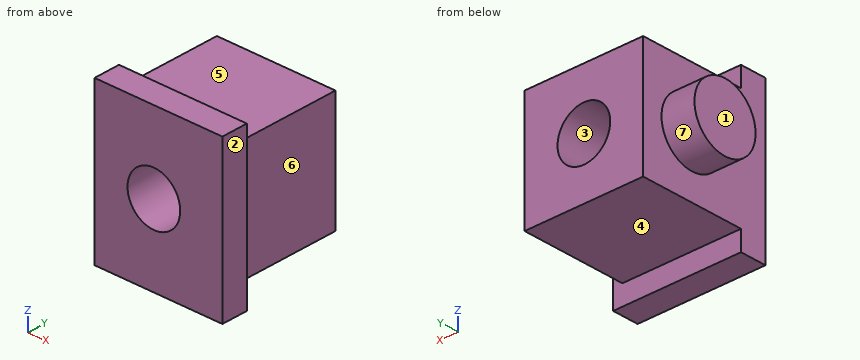
Autodesk Inventor part; units mm, degrees
ref_plane "YZ Plane" through (0, 0, 0) normal (1, 0, 0) x (0, 1, 0)
ref_plane "XZ Plane" through (0, 0, 0) normal (0, 1, 0) x (-1, 0, 0)
ref_plane "XY Plane" through (0, 0, 0) normal (0, 0, 1) x (1, 0, 0)
sketch "Sketch1" plane through (0, 0, 0) normal (0, 1, 0) x (-1, 0, 0)
  line L0 (0, 0) -> (30.1625, 0)
  line L1 (30.1625, 0) -> (30.1625, -31.75)
  line L2 (30.1625, -31.75) -> (0, -31.75)
  line L3 (0, -31.75) -> (0, 0)
  dimension "d0" = 31.75
  dimension "d1" = 30.1625
extrude "Extrusion1" add sketch "Sketch1" along normal blind 31.75
sketch "Sketch2" plane through (-30.1625, 0, 0) normal (0, 0, 1) x (1, 0, 0)
  line L0 (0, 0) -> (0, 31.75)
  line L1 (30.1625, 0) -> (30.1625, 31.75)
  line L2 (30.1625, 0) -> (0, 0)
  line L3 (0, 6.35) -> (30.1625, 6.35)
  line L4 (30.1625, 6.35) -> (30.1625, 31.75)
  line L5 (30.1625, 31.75) -> (0, 31.75)
  line L6 (0, 31.75) -> (0, 6.35)
  dimension "d5" = 6.35
extrude "Extrusion2" cut sketch "Sketch2" against normal blind 1.5875 contours L0 L5 L1 L3
sketch "Sketch3" plane through (0, 0, 0) normal (1, 0, 0) x (0, 0, -1)
  line L0 (1.5875, 31.75) -> (1.5875, 6.35)
  line L1 (31.75, 0) -> (31.75, 31.75)
  line L2 (1.5875, 6.35) -> (31.75, 6.35)
  line L3 (31.75, 6.35) -> (31.75, 31.75)
  line L4 (31.75, 31.75) -> (1.5875, 31.75)
  line L5 (1.5875, 31.75) -> (1.5875, 6.35)
  point P0 (0, 0)
extrude "Extrusion3" cut sketch "Sketch3" against normal blind 1.5875
sketch "Sketch4" plane through (0, 0, -31.75) normal (0, 0, -1) x (-1, 0, 0)
  line L0 (0, 6.35) -> (30.1625, 6.35)
  line L1 (30.1625, 6.35) -> (30.1625, 31.75)
  line L2 (1.5875, 6.35) -> (30.1625, 6.35)
  line L3 (30.1625, 6.35) -> (30.1625, 31.75)
  line L4 (30.1625, 31.75) -> (1.5875, 31.75)
  line L5 (1.5875, 31.75) -> (1.5875, 6.35)
  line L6 (1.5875, 31.75) -> (1.5875, 6.35)
  point P0 (0, 0)
  dimension "d10" = 0
extrude "Extrusion4" cut sketch "Sketch4" against normal blind 1.5875
sketch "Sketch9" plane through (0, 31.75, 0) normal (0, 1, 0) x (1, 0, 0)
  line L0 (0, 31.75) -> (0, 0)
  line L1 (-30.1625, 31.75) -> (0, 31.75)
  point P0 (-15.875, 15.875)
  dimension "d23" = 15.875
  dimension "d24" = 15.875
hole "Hole1" at (-15.875, 31.75, -15.875) direction (0, -1, 0) diameter 12.7 end through all
sketch "Sketch10" plane through (-30.1625, 0, -31.75) normal (-1, 0, 0) x (0, 0, 1)
  circle A0 centre (15.875, 19.05) radius 7.9375
  line L0 (31.75, 0) -> (31.75, 6.35)
  line L1 (1.5875, 31.75) -> (30.1625, 31.75)
  line L2 (30.1625, 6.35) -> (30.1625, 31.75)
  dimension "d33" = 15.875
  dimension "d34" = 15.875
extrude "Extrusion6" add sketch "Sketch10" along normal blind 7.9375
sketch "Sketch12" plane through (0, 0, 0) normal (1, 0, 0) x (0, 0, -1)
  line L0 (31.75, 6.35) -> (0, 6.35)
  line L1 (0, 0) -> (0, 6.35)
  line L2 (31.75, 0) -> (0, 0)
  line L3 (31.75, 0) -> (31.75, 6.35)
extrude "Extrusion8" add sketch "Sketch12" along normal blind 0.635
sketch "Sketch13" plane through (-30.1625, 0, 0) normal (0, 0, 1) x (1, 0, 0)
  line L0 (0, 6.35) -> (30.7975, 6.35)
  line L1 (0, 0) -> (0, 6.35)
  line L2 (30.7975, 0) -> (0, 0)
  line L3 (30.7975, 6.35) -> (30.7975, 0)
  point P0 (30.1625, 0)
extrude "Extrusion9" add sketch "Sketch13" along normal blind 3.175
sketch "Sketch14" plane through (-30.1625, 0, -31.75) normal (0, 0, -1) x (-1, 0, 0)
  line L0 (0, 6.35) -> (-30.7975, 6.35)
  line L1 (-30.7975, 0) -> (-30.7975, 6.35)
  line L2 (0, 0) -> (-30.7975, 0)
  line L3 (0, 0) -> (0, 6.35)
  point P0 (-30.1625, 0)
extrude "Extrusion10" add sketch "Sketch14" along normal blind 3.175
properties part number "WackyPlug"
The model under review builds one solid part; all positions refer to its coordinate system, in mm. Face numbers are marked on the shaded views. A direction names the side the tool comes from. Round coordinates to 2 decimals unless told otherwise and drop trailing zeros.
(1) For P1, Ø2, axis at x = -25, y = 21.5, coming from the +Z side; P2, Ø7.5, axis at y = 18.5, z = -14, coming from the +X side; P3, Ø7.5, axis at x = -20.5, y = 22.5, coming from the -Z side, all flat-tipped, find the tip position at first contact; note any pin that passes through.
Working result:
P1: stops at z = -1.59
P2: stops at x = -1.59
P3: stops at z = -30.16
(2) Mouldability with a two-part tool opening along X and no side actions: class the marked faces 1, 2 and 3 as released by +X, released by -X, zero draft, split by the parting line, or undercut.
Working result:
face 1: released by -X
face 2: released by +X
face 3: undercut
(3) Wall thickness on L1, parallel to X at y = 3, z = -8.5 (1 decimal); L2, parallel to Z at x = -29.5, y = 23: over which ranges is each line inside the solid? List them lowest first.
Working result:
L1: x = -30.2 to 0.6
L2: z = -30.16 to -1.59
(4) Tool access review of the marked faces 4, 5, 6 and 7: name each direction out of +Z, -Z, +X, -X, +Y, -Y from which nothing blocks a thin tool from reaching the whole face with its end or side.
Working result:
face 4: -Z, +X, -X, +Y
face 5: +Z, +X, -X, +Y
face 6: +Z, -Z, +X, +Y
face 7: -X
